The model under review builds one solid part; all positions refer to its coordinate system, in mm. Face numbers are marked on the shaded views. A direction names the side the tool comes from. Coordinates: 2 decimals unless noted, no trailing zeros. Write each loop counter-clockwise with the first axis right and the second up, starting at its lowest first coordinate (ties: lowest second). Pieces come first, ordered by that corner, then holes. Notation, with made-up numbers: M 6,-3.75 L 51,-3.75 A15 cw 51,12.25 Z; hole C -39,9.25 d10. An arc over 180 degrees is marked long. Answer as a JSON object with one key per item and string values.
Autodesk Fusion 360 part; units mm, degrees
sketch "草图1" plane through (0, 0, 0) normal (0, 0, 1) x (1, 0, 0)
  line L0 (29.8435, -2) -> (-30.1565, -2)
  line L1 (-30.1565, -2) -> (-30.1565, 2)
  line L2 (-30.1565, 2) -> (29.8435, 2)
  line L3 (29.8435, 2) -> (29.8435, -2)
  line L4 (-30.1565, 2) -> (-40.7091, 0)
  line L5 (-40.7091, 0) -> (-30.1565, -2)
  point P0 (-0.1565, 0)
  dimension "d1" = 60
  dimension "d2" = 4
extrude "拉伸1" add sketch "草图1" along normal blind 1.2
sketch "草图2" plane through (0, 0, 0) normal (0, 0, 1) x (1, 0, 0)
  circle A0 centre (9, 0) radius 2.36
  dimension "d5" = 4.72
extrude "拉伸2" add sketch "草图2" along normal blind 14.8
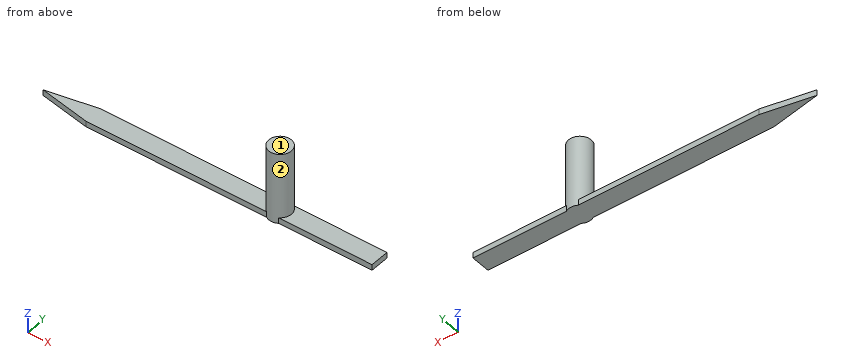
(1) For the marked faces 1 and 2, list the 3-axis set-ups (+Z, -Z, +X, -X, +Y, -Y) from which the entire face can be reached by the end or side of a thin tool; tool diameter is ignored.
Results list:
{"face 1": "+Z, +X, -X, +Y, -Y", "face 2": "+Z"}
(2) Wall thickness on line 1 along Z through (x, y) = (18, -1.85); line 2 along X through (y, z) = (-0.95, 7.25); line 3 along X through (y, z) = (-1.6, 4): over which ranges is each line inside the solid? List them lowest first. Write a range as from..to.
Results list:
{"line 1": "0..1.2", "line 2": "6.84..11.16", "line 3": "7.27..10.73"}
(3) Add section B-B on y = 1.15. Give the boundary of the cut face in (x, z).
Results list:
{"outline": "M -34.64,0 L 29.84,0 L 29.84,1.2 L 11.06,1.2 L 11.06,14.8 L 6.94,14.8 L 6.94,1.2 L -34.64,1.2 Z"}
(4) Add section C-C on z = 4.5. Give the boundary of the cut face in (x, y), and give its area (3 significant figures).
Results list:
{"outline": "C 9,0 d4.72", "area": "17.5 mm²"}
(5) For pin 1 Ø2 at (x, y) = (-12.5, 0.5) entering from +Z; pin 2 Ø8 at (x, z) = (2.5, 5.5) entering from -Y; pin 3 Ø1 at (x, z) = (10, 7.5) entering from +Y; pin 4 Ø1.3 at (x, z) = (16.5, 0.5) entering from -Y, all flat-tipped, find the tip position at first contact; note any pin that passes through.
Results list:
{"pin 1": "z = 1.2", "pin 2": "through", "pin 3": "y = 2.31", "pin 4": "y = -2"}
(6) Add section A-A on x = -8. Give the boundary of the cut face in (y, z), and give its area (3 significant figures).
Results list:
{"outline": "M -2,0 L 2,0 L 2,1.2 L -2,1.2 Z", "area": "4.80 mm²"}
(7) Add section D-D on x = -34. Give the boundary of the cut face in (y, z).
Results list:
{"outline": "M -1.27,0 L 1.27,0 L 1.27,1.2 L -1.27,1.2 Z"}
